```python
from build123d import *

# Parameters (mm, degrees)
BOSS_EXTRUDE1_DEPTH = 60
SKETCH1_3_R         = 7.5
BOSS_EXTRUDE2_DEPTH = 10
SKETCH2_R           = 7.5
CUT_EXTRUDE1_DEPTH  = 123.678441464
FILLET1_RADIUS      = 30
FILLET1_LENGTH      = 10
SKETCH3_R           = 15
CUT_EXTRUDE2_DEPTH  = 127.889565743


with BuildPart() as part:
    # Sketch1 → Boss-Extrude1 (new body)
    with BuildSketch(Plane.XY):
        Polygon((0, 0), (85, 0), (85, 10), (-2.679491924, 10), (-65.621778265, -26.339745962), (-60.621778265, -35), align=None)
    extrude(amount=BOSS_EXTRUDE1_DEPTH)

    # Sketch1<3> → Boss-Extrude2 (add)
    with BuildSketch(Plane.XY):
        with BuildLine():
            Line((6.864064603, 10), (85, 10))
            Line((85, 10), (85, 60))
            ThreePointArc((85, 60), (75.23946894, 74.055175745), (58.660271303, 69.818887568))
            Line((58.660271303, 69.818887568), (6.864064603, 10))
        make_face()
        with Locations((70, 60)):
            Circle(SKETCH1_3_R, mode=Mode.SUBTRACT)
    extrude(amount=BOSS_EXTRUDE2_DEPTH)

    # Sketch2 → Cut-Extrude1 (cut, through all)
    with BuildSketch(Plane(origin=(0, 10, 0), x_dir=(1, 0, 0), z_dir=(0, 1, 0))):
        with Locations(Location((20, -45, 0), (0, 0, 270))):
            Circle(SKETCH2_R)
        with Locations(Location((70, -45, 0), (0, 0, 270))):
            Circle(SKETCH2_R)
    extrude(amount=-CUT_EXTRUDE1_DEPTH, mode=Mode.SUBTRACT)

    # Fillet1: full round fillet: the end face becomes a half cylinder, R = half its width
    fillet1_face = Plane((-63.121778265, -30.669872981, 30), x_dir=(-0.5, 0.866025403784, 0), z_dir=(-0.866025403784, -0.5, 0))  # on the end face: x along it, z out of the body
    fillet1_slab = fillet1_face.offset(-FILLET1_RADIUS / 2) * Box(FILLET1_LENGTH, 2 * FILLET1_RADIUS, FILLET1_RADIUS, mode=Mode.PRIVATE)  # the body's end, R deep
    fillet1_round = Plane((-37.141016151, -15.669872981, 30), x_dir=(-0.866025403784, -0.5, 0), z_dir=(-0.5, 0.866025403784, 0)) * Cylinder(FILLET1_RADIUS, FILLET1_LENGTH, mode=Mode.PRIVATE)  # its axis R under the face
    add(fillet1_slab - fillet1_round, mode=Mode.SUBTRACT)

    # Sketch3 → Cut-Extrude2 (cut, through all)
    with BuildSketch(Plane(origin=(-5, 8.660254038, 0), x_dir=(0.8660254037844345, 0.5000000000000073, 0), z_dir=(-0.5000000000000073, 0.8660254037844345, 0))):
        with Locations(Location((-40, -30, 0), (0, 0, 180))):
            Circle(SKETCH3_R)
    extrude(amount=-CUT_EXTRUDE2_DEPTH, mode=Mode.SUBTRACT)


solid = part.part
```
CAD build for the part. Positions are in the model's coordinates, mm. A direction names the side the tool comes from. Round coordinates to 2 decimals unless told otherwise and drop trailing zeros. Write each loop counter-clockwise with the first axis right and the second up, starting at its lowest first coordinate (ties: lowest second). Pieces come first, ordered by that corner, then holes. Notation, with made-up numbers: (17.5, 25.25) - (23.5, 25.25) arc R5 ccw to (23.5, 34.25) - close; hole circle Ø9 at (-30, 7.5). An arc over 180 degrees is marked (long way). Write item = value, one per line. Start each with the question number.
Q1. Drop flat-ended pins along their axis: pin 1 (17 mm diameter, centred on x = 20, z = 45, fed in from -Y); pin 2 (19.5 mm diameter, centred on x = 46.5, y = 55.5, fed in from +Z); pin 3 (6 mm diameter, centred on y = 55.5, z = 8, fed in from -X). Give the stop position or say it passes through.
Q2. Mould opens along Z. For faces 1 (the flat face through (45, 24, 0)), 2 (the flat face through (42, 0, 30)), 3 (the cylindrical face through (26.324, 5.07, 49.032)), 4 (the cylindrical face through (63.346, 5.07, 48.461)) say: pulls with the +Z half, pulls with the -Z half, needs draft (parallel to the pull), parting line crosses it, or undercut.
Q3. Band-saw the part on D-D (x = 20). Give the cut face in (y, z), then the cut area to 3 significant figures.
Q4. Band-saw the part on B-B (y = 63). Give the cut face in (x, z).
Q5. Which spindle directions (+Z, -Z, +X, -X, +Y, -Y) get a long thin tool onto all of the face, cutting with end or side? Do faces 5 (the cylindrical face through (64.5, 65.1, 4.9)), 6 (the flat face through (54, 36, 10)). Say none if no direction does.
Q6. Band-saw the part on A-A (x = 70). Give the cut face in (y, z).
Q7. Band-saw the part on C-C (z = 23). Give the cut face in (x, y), then the cut area to 3 significant figures.
Q8. Probe L1, parallel to Y at x = 70, z = 3.75; L2, parallel to X at y = 5.5, z = 45; L3, parallel to X at y = 7, z = 45. List the from-to ranges inside material, lowest first. Write a range as from..to.
Answers below:
q1.pin_1 = 0
q1.pin_2 = 10
q1.pin_3 = 43.66
q2.face_1 = pulls with the -Z half
q2.face_2 = needs draft
q2.face_3 = undercut
q2.face_4 = undercut
q3.outline = (0, 0) - (25.17, 0) - (25.17, 10) - (10, 10) - (10, 37.5) - (0, 37.5) - close; (0, 52.5) - (10, 52.5) - (10, 60) - (0, 60) - close
q3.area = 602 mm2
q4.outline = (52.76, 0) - (63.13, 0) - (63.13, 10) - (52.76, 10) - close; (76.87, 0) - (84.7, 0) - (84.7, 10) - (76.87, 10) - close
q5.face_5 = +Z, -Z
q5.face_6 = +Z, +X, -X, +Y
q6.outline = (0, 0) - (52.5, 0) - (52.5, 10) - (10, 10) - (10, 37.5) - (0, 37.5) - close; (0, 52.5) - (10, 52.5) - (10, 60) - (0, 60) - close; (67.5, 0) - (75, 0) - (75, 10) - (67.5, 10) - close
q7.outline = (-64.9, -25.93) - (-59.9, -34.59) - (-46.13, -26.63) - (-51.13, -17.97) - close; (-28.15, -4.71) - (-23.15, -13.37) - (0, 0) - (85, 0) - (85, 10) - (-2.68, 10) - close
q7.area = 1,300 mm2
q8.L1 = 0..52.5, 67.5..75
q8.L2 = -10.47..12.5, 27.5..62.5, 77.5..85
q8.L3 = -7.88..12.5, 27.5..62.5, 77.5..85
